```python
from build123d import *

# Parameters (mm, degrees)
SKETCH1_W           = 77.5208
SKETCH1_H           = 79.883
BOSS_EXTRUDE1_DEPTH = 36.0172
SKETCH4_R           = 3.5687
BOSS_EXTRUDE2_DEPTH = 9.5758
SKETCH5_R           = 3.5687
BOSS_EXTRUDE3_DEPTH = 9.5758
SKETCH6_R           = 1.3462
CUT_EXTRUDE1_DEPTH  = 8.636


with BuildPart() as part:
    # Sketch1 → Boss-Extrude1 (new body)
    with BuildSketch(Plane.XY):
        with Locations((38.7604, 39.9415)):
            Rectangle(SKETCH1_W, SKETCH1_H)
    extrude(amount=BOSS_EXTRUDE1_DEPTH)

    # Sketch4 → Boss-Extrude2 (add)
    with BuildSketch(Plane(origin=(0, 0, 0), x_dir=(-1, 0, 0), z_dir=(0, 0, -1))):
        with Locations(Location((-71.1708, 2.54, 0), (0, 0, 225.376971118))):
            Circle(SKETCH4_R)
        with Locations(Location((-3.0734, 2.452500211, 0), (0, 0, 223.410850824))):
            Circle(SKETCH4_R)
    extrude(amount=BOSS_EXTRUDE2_DEPTH)

    # Sketch5 → Boss-Extrude3 (add)
    with BuildSketch(Plane(origin=(0, 0, 0), x_dir=(-1, 0, 0), z_dir=(0, 0, -1))):
        with Locations(Location((-10.7188, 77.343, 0), (0, 0, 134.623028882))):
            Circle(SKETCH5_R)
        with Locations(Location((-64.0588, 76.835, 0), (0, 0, 121.340374815))):
            Circle(SKETCH5_R)
    extrude(amount=BOSS_EXTRUDE3_DEPTH)

    # Sketch6 → Cut-Extrude1 (cut)
    with BuildSketch(Plane(origin=(0, 0, -9.5758), x_dir=(-1, 0, 0), z_dir=(0, 0, -1))):
        with Locations((-71.1708, 2.54)):
            Circle(SKETCH6_R)
        with Locations((-3.0734, 2.452500211)):
            Circle(SKETCH6_R)
        with Locations((-10.7188, 77.343)):
            Circle(SKETCH6_R)
        with Locations((-64.0588, 76.835)):
            Circle(SKETCH6_R)
    extrude(amount=-CUT_EXTRUDE1_DEPTH, mode=Mode.SUBTRACT)


solid = part.part
```
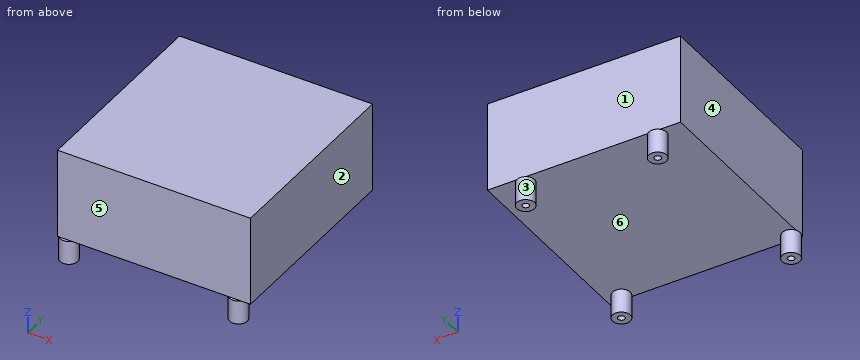
Here's how the part is built. I have some questions about the finished solid (model axes, mm). Face numbers are marked on the shaded views. A direction names the side the tool comes from. Coordinates: 2 decimals unless noted, no trailing zeros. Loops run counter-clockwise (first coordinate to the right, second up) from the corner with the lowest first, then second, coordinate; pieces in that order, holes last. Notation, with made-up numbers: (-21, -34.5) - (-14, -34.5) arc R9 cw to (-14, -20.5) - close; hole circle Ø4 at (5.5, -2.75). An arc over 180 degrees is marked (long way). Return JSON: item names as keys, results as strings. Group by question number.
Item 1: On a 3-axis mill with a long thin cutter (end or side, diameter ignored), from which of +Z, -Z, +X, -X, +Y, -Y can I reach the whole of each face in a straight line? I mean the marked faces 1, 2 and 3. Say none if no direction works.
Item 2: We'd pull the mould along X, two halves only. Please class the marked faces 4, 5 and 6: +X half, -X half, draft (parallel to the pull), parting line (faces both ways), or undercut.
Item 3: If we section it at A-A on x = 50: Write out the boundary of the cut face in (y, z), and give its area (3 significant figures).
Item 4: Will these pins go through, and if not, where does the flat tip stop? P1, Ø5, axis at y = 52, z = 24, coming from the -X side; P2, Ø5, axis at x = 32, z = -1.5, coming from the -Y side; P3, Ø2, axis at x = 10.72, y = 77.34, coming from the -Z side.
Item 5: If we section it at B-B on z = 28.5: Write out the boundary of the cut face in (x, y).
Item 6: I need wall thicknesses on line 1 (Y direction, x = 10.5, z = -4.5); line 2 (Z direction, x = 36, y = 25.5); line 3 (Y direction, x = 53.5, z = 21). Which ranges of each line are inside material? Lowest first, please. Write a range as from..to.
Calculated:
{
 "1": {"face 1": "+Z, +X, -X, +Y", "face 2": "+Z, -Z, +X, +Y, -Y", "face 3": "-Z"},
 "2": {"face 4": "-X half", "face 5": "draft", "face 6": "undercut"},
 "3": {"outline": "(0, 0) - (79.88, 0) - (79.88, 36.02) - (0, 36.02) - close", "area": "2,880 mm^2"},
 "4": {"P1": "stops at x = 0", "P2": "stops at y = 0", "P3": "stops at z = -0.94"},
 "5": {"outline": "(0, 0) - (77.52, 0) - (77.52, 79.88) - (0, 79.88) - close"},
 "6": {"line 1": "y = 73.78..76.01, 78.67..80.9", "line 2": "z = 0..36.02", "line 3": "y = 0..79.88"}
}
